Autodesk Inventor part; units mm, degrees
ref_plane "YZ Plane" through (0, 0, 0) normal (1, 0, 0) x (0, 1, 0)
ref_plane "XZ Plane" through (0, 0, 0) normal (0, 1, 0) x (-1, 0, 0)
ref_plane "XY Plane" through (0, 0, 0) normal (0, 0, 1) x (1, 0, 0)
sketch "Sketch2" plane through (0, 0, 0) normal (0, 0, 1) x (1, 0, 0)
  line L0 (0, 277.6336) -> (196.3166, 196.3166) construction
  line L1 (196.3166, 196.3166) -> (277.6336, 0) construction
  line L2 (277.6336, 0) -> (196.3166, -196.3166) construction
  line L3 (196.3166, -196.3166) -> (0, -277.6336) construction
  line L4 (0, -277.6336) -> (-196.3166, -196.3166) construction
  line L5 (-196.3166, -196.3166) -> (-277.6336, 0) construction
  line L6 (-277.6336, 0) -> (-196.3166, 196.3166) construction
  line L7 (-196.3166, 196.3166) -> (0, 277.6336) construction
  line L8 (-196.3166, 196.3166) -> (0, 277.6336) construction
  line L9 (-461.2666, 773.8898) -> (-221.0579, 873.3874) construction
  line L10 (-98.1583, 236.9751) -> (-341.1623, 823.6386) construction
  line L11 (-221.0579, 873.3874) -> (0, 873.3874) construction
  line L12 (0, 873.3874) -> (0, 277.6336) construction
  line L13 (-461.2666, 773.8898) -> (-617.5782, 617.5782) construction
  line L14 (-617.5782, 617.5782) -> (-196.3166, 196.3166) construction
  line L15 (-5, 280.9745) -> (-195.1434, 202.2145) construction
  line L16 (-195.1434, 202.2145) -> (-610.5071, 617.5782) construction
  line L17 (-610.5071, 617.5782) -> (-458.4343, 769.651) construction
  line L18 (-458.4343, 769.651) -> (-220.0634, 868.3874) construction
  line L19 (-220.0634, 868.3874) -> (-5, 868.3874) construction
  line L20 (-5, 868.3874) -> (-5, 280.9745) construction
  line L21 (-13, 286.3199) -> (-193.2664, 211.6511) construction
  line L22 (-193.2664, 211.6511) -> (-599.1934, 617.5782) construction
  line L23 (-599.1934, 617.5782) -> (-453.9027, 762.8689) construction
  line L24 (-453.9027, 762.8689) -> (-218.4721, 860.3874) construction
  line L25 (-218.4721, 860.3874) -> (-13, 860.3874) construction
  line L26 (-13, 860.3874) -> (-13, 286.3199) construction
  line L27 (-5, 280.9745) -> (-195.1434, 202.2145)
  line L28 (-195.1434, 202.2145) -> (-193.2664, 211.6511)
  line L29 (-193.2664, 211.6511) -> (-13, 286.3199)
  line L30 (-13, 286.3199) -> (-5, 280.9745)
  point P0 (0, 0)
  point P1 (0, 0)
  point P2 (0, 0)
  dimension "d0" = 513
  dimension "d1" = 260
  dimension "d2" = 635
  dimension "d6" = 5
  dimension "d7" = 8
extrude "Extrusion1" add sketch "Sketch2" along normal mid plane 80
sketch "Sketch3" plane through (-13, 286.3199, -40) normal (-0.3827, 0.9239, 0) x (0.9239, 0.3827, 0)
  line L0 (-165.0595, -15) -> (-30.0595, -15)
  line L1 (-30.0595, -15) -> (-30.0595, -65)
  line L2 (-30.0595, -65) -> (-165.0595, -65)
  line L3 (-165.0595, -65) -> (-165.0595, -15)
  circle A0 centre (-15.0595, -40) radius 5
  circle A1 centre (-180.0595, -40) radius 5
  line L4 (0, -80) -> (-195.1189, -80)
  line L5 (-97.5595, -40) -> (-97.5595, -80) construction
  line L6 (5.3454, 0) -> (5.3454, -80) construction
  point P0 (-97.5595, -15)
  point P1 (-165.0595, -40)
  point P2 (-30.0595, -40)
  point P3 (5.3454, -40)
  dimension "d10" = 135
  dimension "d11" = 10
  dimension "d12" = 15
  dimension "d13" = 50
extrude "Extrusion2" cut sketch "Sketch3" against normal up to surface (8 mm away)
fillet "Fillet1" radius 5 4 edges at (-163.9643, 219.4589, -25) (-39.2406, 271.1211, -25) (-39.2406, 271.1211, 25) (-163.9643, 219.4589, 25)
equation "\"d0\" = Барабан_габарит_по_кассетам"
equation "\"d1\" = Кассета_длина_грани"
equation "\"d2\" = Кассета_высота"
equation "\"d10\" = Барабан_Длина_окна"
equation "\"d11\" = Кассета_Диам_шпильки"
equation "\"d13\" = Барабан_Ширина_окна"
properties part number "ДМФ 01 54 Нижний лист"
Verification items for the finished model (mm, model axes). A direction names the side the tool comes from. Round coordinates to 2 decimals unless told otherwise and drop trailing zeros. Write each loop counter-clockwise with the first axis right and the second up, starting at its lowest first coordinate (ties: lowest second). Pieces come first, ordered by that corner, then holes.
1. Section check C-C on z = -3. Enter the section's corners in (x, y), plus the area to 3 significant figures.
2. Section check D-D on z = 32. Enter the section's corners in (x, y), plus the area to 3 significant figures.
3. Scan lines: L1, parallel to Z at x = -64, y = 260; L2, parallel to Y at x = -169.5, z = 5.5; L3, parallel to Y at x = -18.5, z = 32. Record each from-to range of solid material in increasing order.
4. Access from +Z, -Z, +X, -X, +Y, -Y to the whole of each face (thin tool, end or side, straight path). Record for faces 4 (the cylindrical face through (-40.608, 270.494, -23.574)), 5 (the flat face through (-163.986, 219.511, 0.28)), 6 (the flat face through (-98.741, 242.146, -27.227)).
5. Gauge pin test, flat ends, axial feed: P1, Ø1.5, axis at x = -136, z = 31.5, coming from the -Y side; P2, Ø12, axis at x = -79, z = 29, coming from the -Y side; P3, Ø2, axis at y = 220.5, z = 28, coming from the +X side. Record the tip position at first contact, or that the pin passes through.
6. Section check B-B on x = -121.5. Enter the section's corners in (y, z).
7. Section check A-A on y = 230. Enter the section's corners in (x, z).
8. Draft check along X on faces 1 (the cylindrical face through (-173.58, 215.54, 1.92)), 2 (the flat face through (-9.056, 283.685, -0.56)), 3 (the cylindrical face through (-40.54, 270.52, 23.5)). Enter one of: +X half, -X half, draft (parallel to the pull), parting line (faces both ways), or undercut.
Answer:
1. outline: (-195.14, 202.21) - (-179.99, 208.49) - (-183.05, 215.88) - (-193.27, 211.65) - close; (-175.66, 218.94) - (-172.6, 211.55) - (-162.43, 215.76) - (-165.5, 223.15) - close; (-40.77, 274.82) - (-37.71, 267.43) - (-27.55, 271.64) - (-30.61, 279.03) - close; (-23.22, 282.09) - (-20.16, 274.7) - (-5, 280.97) - (-13, 286.32) - close
1. area: 396 mm2
2. outline: (-195.14, 202.21) - (-5, 280.97) - (-13, 286.32) - (-193.27, 211.65) - close
2. area: 1,600 mm2
3. L1: z = -40 to -25, 25 to 40
3. L2: y = 212.84 to 221.5
3. L3: y = 275.38 to 284.04
4. face 4: -X, -Y
4. face 5: +X, +Y
4. face 6: +Z, -Z, +X, -Y
5. P1: stops at y = 226.4
5. P2: stops at y = 247.84
5. P3: stops at x = -148.58
6. outline: (232.72, -40) - (241.38, -40) - (241.38, -25) - (232.72, -25) - close; (232.72, 25) - (241.38, 25) - (241.38, 40) - (232.72, 40) - close
7. outline: (-148.97, -40) - (-128.06, -40) - (-128.06, -25) - (-148.97, -25) - close; (-148.97, 25) - (-128.06, 25) - (-128.06, 40) - (-148.97, 40) - close
8. face 1: undercut
8. face 2: +X half
8. face 3: -X half
